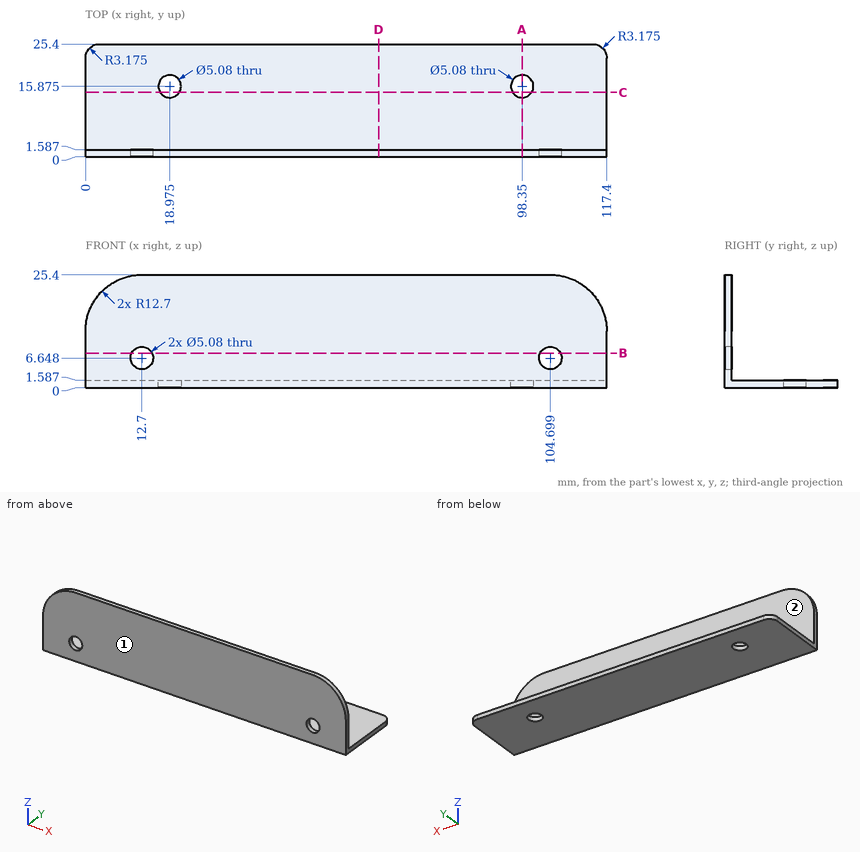
Answer from the drawing. Dimensions are ordinates in mm from the lowest x, y and z of the part. A direction names the side the tool comes from. Round coordinates to 2 decimals unless told otherwise and drop trailing zeros. Loops run counter-clockwise (first coordinate to the right, second up) from the corner with the lowest first, then second, coordinate; pieces in that order, holes last. Notation, with made-up numbers: (57, -16) - (85, -16) arc R33 ccw to (85, 19) - close; hole circle Ø1 at (-10, 70). An arc over 180 degrees is marked (long way). Return JSON: item names as keys, results as strings. Group by question number.
1. The part is cut by section B-B on z = 7.75. Determine the outline of the cut face in (x, y), then the cut area to 3 significant figures.
2. The part is cut by section C-C on y = 14.5. Determine the outline of the cut face in (x, z) (1 decimal), then the cut area to 3 significant figures.
3. The part is cut by section A-A on x = 98.35. Determine the outline of the cut face in (y, z) (1 decimal).
4. Which of the six approach directions +Z, -Z, +X, -X, +Y, -Y give full straight-line access (tool end or side, diameter ignored) to the marked faces 1 and 2?
5. The part is cut by section D-D on x = 66. Determine the outline of the cut face in (y, z).
6. Each of these flat-tipped pins is pushed along its axis until it touches: P1, Ø1.5, axis at x = 101, y = 17.5, coming from the +Z side; P2, Ø4, axis at x = 12.7, z = 6.65, coming from the +Y side; P3, Ø1, axis at x = 31.5, z = 11, coming from the +Y side. Where does it stop, or does it pass through?
7. Consider probe 1 along Y at (x, z) = (86, 10.5). Determine where the line is inside the solid, lowest interval first.
Resolved:
{
 "1": {"outline": "(0, 0) - (10.41, 0) - (10.41, 1.59) - (0, 1.59) - close; (14.99, 0) - (102.41, 0) - (102.41, 1.59) - (14.99, 1.59) - close; (106.99, 0) - (117.4, 0) - (117.4, 1.59) - (106.99, 1.59) - close", "area": "172 mm²"},
 "2": {"outline": "(0, 0) - (16.8, 0) - (16.8, 1.6) - (0, 1.6) - close; (21.1, 0) - (96.2, 0) - (96.2, 1.6) - (21.1, 1.6) - close; (100.5, 0) - (117.4, 0) - (117.4, 1.6) - (100.5, 1.6) - close", "area": "173 mm²"},
 "3": {"outline": "(0, 0) - (13.3, 0) - (13.3, 1.6) - (1.6, 1.6) - (1.6, 25.4) - (0, 25.4) - close; (18.4, 0) - (25.4, 0) - (25.4, 1.6) - (18.4, 1.6) - close"},
 "4": {"face 1": "+Z, -Z, +X, -X, -Y", "face 2": "+Z, +X, -X, +Y"},
 "5": {"outline": "(0, 0) - (25.4, 0) - (25.4, 1.59) - (1.59, 1.59) - (1.59, 25.4) - (0, 25.4) - close"},
 "6": {"P1": "stops at z = 1.59", "P2": "passes through", "P3": "stops at y = 1.59"},
 "7": {"probe 1": "y = 0 to 1.59"}
}
